```python
from build123d import *
from OCP.BRepFilletAPI import BRepFilletAPI_MakeChamfer

# Parameters (mm, degrees)
BOSS_EXTRUDE1_DEPTH = 20
CHAMFER1_SIZE       = 1.2
CHAMFER1_SIZE2      = 0.321539031
CHAMFER2_SIZE       = 3
CHAMFER2_SIZE2      = 2.100622615


# Read off the part's stored shape, not the designer's step: Revolve1
with BuildPart() as part:
    # Sketch1 → Boss-Extrude1 (new body)
    with BuildSketch(Plane(origin=(0, 0, 0), x_dir=(1, 0, 0), z_dir=(0, 1, 0))):
        with BuildLine():
            Line((-1.537530488, -1.67), (1.537530488, -1.67))
            ThreePointArc((1.537530488, -1.67), (0, 2.27), (-1.537530488, -1.67))
        make_face()
    extrude(amount=BOSS_EXTRUDE1_DEPTH)

    # Chamfer1: one chamfer whose edges measure the first distance from different faces: ONE call of the kernel's chamfer builder (chamfer() names one face for all edges)
    chamfer1_edges_1 = [part.edges().sort_by_distance(p)[0] for p in [
        (0, 20, -2.27),
    ]]
    chamfer1_side_1 = [part.faces().sort_by_distance(p)[0] for p in [
        (0, 10, -2.27),
    ]]
    chamfer1_edges_2 = [part.edges().sort_by_distance(p)[0] for p in [
        (0, 20, 1.67),
    ]]
    chamfer1_side_2 = [part.faces().sort_by_distance(p)[0] for p in [
        (0, 10, 1.67),
    ]]
    chamfer1 = BRepFilletAPI_MakeChamfer(part.part.solid().wrapped)
    for e in chamfer1_edges_1:
        chamfer1.Add(CHAMFER1_SIZE, CHAMFER1_SIZE2, e.wrapped, chamfer1_side_1[0].wrapped)  # the first distance lies on this face
    for e in chamfer1_edges_2:
        chamfer1.Add(CHAMFER1_SIZE, CHAMFER1_SIZE2, e.wrapped, chamfer1_side_2[0].wrapped)  # the first distance lies on this face
    add(Compound.cast(chamfer1.Shape()), mode=Mode.REPLACE)

    # Revolve1 outline → Revolve1 (revolve)
    with BuildSketch(Plane.XY.offset(-0.223266571)):
        with BuildLine():
            Line((6.893266571, 2), (1.893266571, 2))
            Line((1.893266571, 2), (1.893266571, 0))
            Line((1.893266571, 0), (0, 0))
            Line((0, 0), (0, -10))
            Line((0, -10), (6.893266571, -10))
            add(Edge.make_bspline(
                [(6.893266571, -10), (6.893266571, -0.153248468), (2.676005531, -20.148158745), (2.676005531, 12.148158745), (6.893266571, -7.846751532), (6.893266571, 2)],
                knots=[0.057927251, 0.057927251, 0.057927251, 0.057927251, 0.057927251, 0.057927251, 1.057927251, 1.057927251, 1.057927251, 1.057927251, 1.057927251, 1.057927251], degree=5))
        make_face()
    revolve(axis=Axis((0, 0, -0.223266571), (0, 1, 0)))

    # Chamfer2: one chamfer whose edges measure the first distance from different faces: ONE call of the kernel's chamfer builder (chamfer() names one face for all edges)
    chamfer2_edges_1 = [part.edges().sort_by_distance(p)[0] for p in [
        (0, 2, 1.67),
    ]]
    chamfer2_side_1 = [part.faces().sort_by_distance(p)[0] for p in [
        (0, 10.4, 1.67),
    ]]
    chamfer2_edges_2 = [part.edges().sort_by_distance(p)[0] for p in [
        (0, 2, -2.27),
    ]]
    chamfer2_side_2 = [part.faces().sort_by_distance(p)[0] for p in [
        (0, 10.4, -2.27),
    ]]
    chamfer2 = BRepFilletAPI_MakeChamfer(part.part.solid().wrapped)
    for e in chamfer2_edges_1:
        chamfer2.Add(CHAMFER2_SIZE, CHAMFER2_SIZE2, e.wrapped, chamfer2_side_1[0].wrapped)  # the first distance lies on this face
    for e in chamfer2_edges_2:
        chamfer2.Add(CHAMFER2_SIZE, CHAMFER2_SIZE2, e.wrapped, chamfer2_side_2[0].wrapped)  # the first distance lies on this face
    add(Compound.cast(chamfer2.Shape()), mode=Mode.REPLACE)


solid = part.part
```
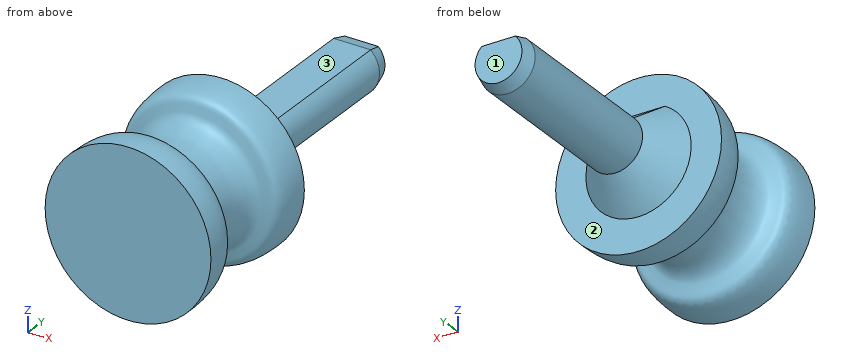
Build history of the part. All positions in model axes, mm. Face numbers are marked on the shaded views. A direction names the side the tool comes from. Give positions to 0.01 mm unless a question says otherwise; leave off trailing zeros. Order: outer loops, then holes, each group sorted by start corner. A loop starts at its lowest first (then second) coordinate and runs counter-clockwise, first axis right, second up. Notation, with made-up numbers: M 31,15.25 L 85,15.25 A23 cw 85,43.25 Z; hole C 43,88.25 d3. An arc over 180 degrees is marked long. Write item = value, one per line. Start each with the question number.
(1) Probe L1, parallel to Y at x = -4.5, z = -4; L2, parallel to Y at x = 5.5, z = -1.25; L3, parallel to Z at x = 5.5, y = 0.5. List the from-to ranges inside material, lowest first. Write a range as [from, to].
(2) Slice it at B-B on y = 2.5. Write the cut outline in (x, z).
(3) Slice it at A-A on y = 13.5. Write the cut outline in (x, z), plus the area to 3 significant figures.
(4) Pin check, flat tips, straight feed: pin 1 Ø1.5 at (x, y) = (3, 3.5) entering from +Z; pin 2 Ø0.9 at (x, y) = (-0.5, 9) entering from +Z; pin 3 Ø2 at (x, y) = (0, 4) entering from -Z. Stop position of each tip, or through.
(5) Which spindle directions (+Z, -Z, +X, -X, +Y, -Y) get a long thin tool onto all of the face, cutting with end or side? Do the marked faces 1, 2 and 3. Say none if no direction does.
Responses:
q1.L1 = [-10, -6.91], [-1.09, 2]
q1.L2 = [-10, -6.85], [-1.15, 2]
q1.L3 = [-4.28, 3.84]
q2.outline = M -2.11,3.42 A4.02 ccw long 2.11,3.42 Z
q3.outline = M -1.54,1.67 A2.27 ccw long 1.54,1.67 Z
q3.area = 14.9 mm2
q4.pin_1 = 2.74
q4.pin_2 = 1.67
q4.pin_3 = -3.67
q5.face_1 = +Z, -Z, +X, -X, +Y
q5.face_2 = +Y
q5.face_3 = +Z, +X, -X, +Y
